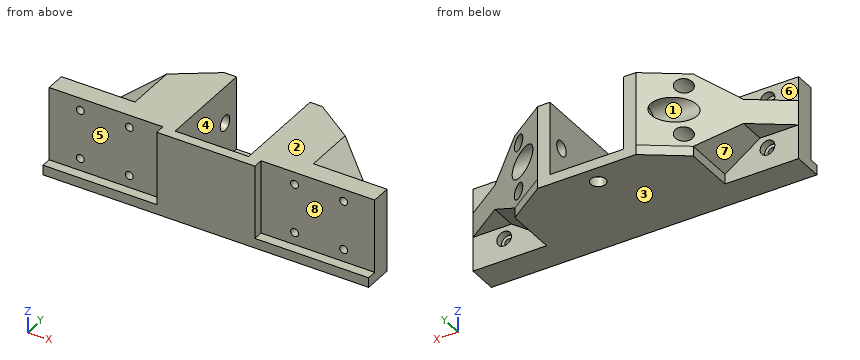
from build123d import *

# Parameters (mm, degrees)
SKETCH1_W               = 132.8
SKETCH1_H               = 44
BOSS_EXTRUDE1_DEPTH     = 4
SKETCH2_W               = 46.4
SKETCH2_H               = 8
BOSS_EXTRUDE2_DEPTH     = 30
BOSS_EXTRUDE3_DEPTH     = 15
CUT_EXTRUDE3_DEPTH      = 91.917325082
CUT_EXTRUDE3_DEPTH_BACK = 91.917325082
SKETCH6_R               = 3.1
SKETCH8_R               = 5.125
CUT_EXTRUDE5_DEPTH      = 96.419914064
SKETCH9_R               = 5.125
CUT_EXTRUDE6_DEPTH      = 96.419914064
CUT_EXTRUDE4_DEPTH      = 82.172409106
SKETCH3_R               = 1.6
CUT_EXTRUDE1_DEPTH      = 30
CUT_EXTRUDE2_DEPTH      = 82.172409106
CUT_EXTRUDE2_DEPTH_BACK = 3
SKETCH4_R               = 3
CUT_EXTRUDE7_DEPTH      = 77.11149716
SKETCH11_R              = 3.1
CUT_EXTRUDE8_DEPTH      = 77.11149716


with BuildPart() as part:
    # Sketch1 → Boss-Extrude1 (new body)
    with BuildSketch(Plane.XY):
        Rectangle(SKETCH1_W, SKETCH1_H)
    extrude(amount=BOSS_EXTRUDE1_DEPTH)

    # Sketch2 → Boss-Extrude2 (add)
    with BuildSketch(Plane.XY.offset(4)):
        with Locations((-43.2, -14)):
            Rectangle(SKETCH2_W, SKETCH2_H)
        Polygon((15, -18), (-15, -18), (-15, 22), (-20, 22), (-20, -10), (-20, -18), (-20, -22), (20, -22), (20, -18), (20, -10), (20, 22), (15, 22), align=None)
        with Locations((43.2, -14)):
            Rectangle(SKETCH2_W, SKETCH2_H)
    extrude(amount=BOSS_EXTRUDE2_DEPTH)

    # Sketch5 → Boss-Extrude3 (add, symmetric)
    with BuildSketch(Plane.XY.offset(19)):
        Polygon((20, -10), (66.4, -10), (20, 22), align=None)
        Polygon((-20, 22), (-20, -10), (-66.4, -10), align=None)
    extrude(amount=BOSS_EXTRUDE3_DEPTH, both=True)

    # Sketch6 → Cut-Extrude3 (cut, two sides: drawn at the far end of the back side and taken through both)
    with BuildSketch(Plane(origin=(-15, 0, 0), x_dir=(0, 0, -1), z_dir=(1, 0, 0)).offset(-CUT_EXTRUDE3_DEPTH_BACK)):
        with Locations(Location((-19, 14.5, 0), (0, 0, 90))):
            Circle(SKETCH6_R)
    extrude(amount=CUT_EXTRUDE3_DEPTH + CUT_EXTRUDE3_DEPTH_BACK, mode=Mode.SUBTRACT)

    # Sketch8 → Cut-Extrude5 (cut, through all)
    with BuildSketch(Plane(origin=(20, 0, 0), x_dir=(0, 0, -1), z_dir=(1, 0, 0))):
        with Locations(Location((-19, 14.5, 0), (0, 0, 90))):
            Circle(SKETCH8_R)
    extrude(amount=CUT_EXTRUDE5_DEPTH, mode=Mode.SUBTRACT)

    # Sketch9 → Cut-Extrude6 (cut, through all)
    with BuildSketch(Plane.ZY.offset(20)):
        with Locations(Location((19, 14.5, 0), (0, 0, 90))):
            Circle(SKETCH9_R)
    extrude(amount=CUT_EXTRUDE6_DEPTH, mode=Mode.SUBTRACT)

    # Sketch7 → Cut-Extrude4 (cut, through all)
    with BuildSketch(Plane(origin=(0, -10, 0), x_dir=(1, 0, 0), z_dir=(0, 1, 0))):
        Polygon((50.681480067, -14), (66.4, -14), (66.4, -4), (36.4, -4), align=None)
        Polygon((66.4, -34), (66.4, -24), (50.681480067, -24), (36.4, -34), align=None)
        Polygon((-66.4, -4), (-66.4, -14), (-50.681480067, -14), (-36.4, -4), align=None)
        Polygon((-50.681480067, -24), (-66.4, -24), (-66.4, -34), (-36.4, -34), align=None)
    extrude(amount=CUT_EXTRUDE4_DEPTH, mode=Mode.SUBTRACT)

    # Sketch3 → Cut-Extrude1 (cut)
    with BuildSketch(Plane(origin=(0, -10, 0), x_dir=(1, 0, 0), z_dir=(0, 1, 0))):
        with Locations(Location((-53.7, -9, 0), (0, 0, 270))):
            Circle(SKETCH3_R)
        with Locations(Location((-33.7, -29, 0), (0, 0, 270))):
            Circle(SKETCH3_R)
        with Locations(Location((-33.7, -9, 0), (0, 0, 270))):
            Circle(SKETCH3_R)
        with Locations(Location((-53.7, -29, 0), (0, 0, 270))):
            Circle(SKETCH3_R)
        with Locations(Location((33.7, -9, 0), (0, 0, 270))):
            Circle(SKETCH3_R)
        with Locations(Location((33.7, -29, 0), (0, 0, 270))):
            Circle(SKETCH3_R)
        with Locations(Location((53.7, -29, 0), (0, 0, 270))):
            Circle(SKETCH3_R)
        with Locations(Location((53.7, -9, 0), (0, 0, 270))):
            Circle(SKETCH3_R)
    extrude(amount=-CUT_EXTRUDE1_DEPTH, mode=Mode.SUBTRACT)

    # Sketch4 → Cut-Extrude2 (cut, two sides: drawn at the far end of the back side and taken through both)
    with BuildSketch(Plane(origin=(0, -10, 0), x_dir=(1, 0, 0), z_dir=(0, 1, 0)).offset(-CUT_EXTRUDE2_DEPTH_BACK)):
        with Locations(Location((-53.7, -9, 0), (0, 0, 90))):
            Circle(SKETCH4_R)
        with Locations(Location((-33.7, -9, 0), (0, 0, 180))):
            Circle(SKETCH4_R)
        with Locations(Location((-33.7, -29, 0), (0, 0, 180))):
            Circle(SKETCH4_R)
        with Locations(Location((-53.7, -29, 0), (0, 0, 270))):
            Circle(SKETCH4_R)
        with Locations((33.7, -9)):
            Circle(SKETCH4_R)
        with Locations(Location((53.7, -9, 0), (0, 0, 90))):
            Circle(SKETCH4_R)
        with Locations(Location((53.7, -29, 0), (0, 0, 90))):
            Circle(SKETCH4_R)
        with Locations((33.7, -29)):
            Circle(SKETCH4_R)
    extrude(amount=CUT_EXTRUDE2_DEPTH + CUT_EXTRUDE2_DEPTH_BACK, mode=Mode.SUBTRACT)

    # Sketch10 → Cut-Extrude7 (cut, through all)
    with BuildSketch(Plane.XY.offset(4)):
        Polygon((20, 22), (36.4, 10.689655172), (36.4, -10), (66.4, -10), (66.4, 22), align=None)
        Polygon((-66.4, 22), (-20, 22), (-36.4, 10.689655172), (-36.4, -10), (-66.4, -10), align=None)
    extrude(amount=-CUT_EXTRUDE7_DEPTH, mode=Mode.SUBTRACT)

    # Sketch11 → Cut-Extrude8 (cut, through all)
    with BuildSketch(Plane.XY.offset(4)):
        with Locations((0, 14.5)):
            Circle(SKETCH11_R)
    extrude(amount=-CUT_EXTRUDE8_DEPTH, mode=Mode.SUBTRACT)


solid = part.part
Source: CAD feature listing. Evaluate the final solid. Frame: model axes, mm. Face numbers are marked on the shaded views. A direction names the side the tool comes from. Coordinates: 2 decimals unless noted, no trailing zeros. Write each loop counter-clockwise with the first axis right and the second up, starting at its lowest first coordinate (ties: lowest second). Pieces come first, ordered by that corner, then holes. Notation, with made-up numbers: M 42.25,-22.75 L 67.25,-22.75 A24 ccw 67.25,11.25 Z; hole C 38,58 d9. An arc over 180 degrees is marked long. Use a Markdown table: item, result.
1) Mould query, pull axis Z, two halves, no side actions, for the marked faces 1, 2, 3 and 4. Classes: pulls with the +Z half, pulls with the -Z half, needs draft (parallel to the pull), parting line crosses it, or undercut.
Conclusion:
| item | result |
|---|---|
| face 1 | undercut |
| face 2 | pulls with the +Z half |
| face 3 | pulls with the -Z half |
| face 4 | needs draft |
2) First-contact query: pin 1 Ø3 at (y, z) = (16.5, 4) entering from -X; pin 2 Ø3.5 at (x, z) = (-33.7, 9) entering from -Y; pin 3 Ø1.8 at (x, z) = (33, 8) entering from +Y. Flat tips, straight axial feed; report the tip coordinate or a pass-through.
Conclusion:
| item | result |
|---|---|
| pin 1 | stops at x = -30.15 |
| pin 2 | stops at y = -18 |
| pin 3 | stops at y = -13 |
3) Section B-B, the plane y = -4.5. Output: boundary loops of the cut face in (x, z) (3 decimals), then the cut area to 3 significant figures.
Conclusion:
| item | result |
|---|---|
| outline | M -58.425,14 L -50.681,14 L -36.4,4 L -36.4,0 L 36.4,0 L 36.4,4 L 50.681,14 L 58.425,14 L 58.425,24 L 50.681,24 L 36.4,34 L 15,34 L 15,4 L -15,4 L -15,34 L -36.4,34 L -50.681,24 L -58.425,24 Z; hole C -33.7,9 d6; hole C -33.7,29 d6; hole C 33.7,9 d6; hole C 33.7,29 d6 |
| area | 2,190 mm^2 |
4) Section D-D, the plane z = 29. Give the number of separate pieces and of enclosed holes in the cut face, then the cut area to 3 significant figures.
Conclusion:
| item | result |
|---|---|
| separate pieces | 5 |
| enclosed holes | 0 |
| area | 2,020 mm^2 |
5) Reachability of the marked faces 5, 6, 7 and 8 from +Z, -Z, +X, -X, +Y, -Y: full face, straight path, thin tool, end or side. Return the list, or none.
Conclusion:
| item | result |
|---|---|
| face 5 | +Z, -X, -Y |
| face 6 | +Z, -X, +Y |
| face 7 | -Z, -X, +Y |
| face 8 | +Z, +X, -Y |
6) Section C-C, the plane x = -53.7. Output: boundary loops of the cut face in (y, z), then the cut area to 3 significant figures.
Conclusion:
| item | result |
|---|---|
| outline | M -22,0 L -10,0 L -10,6 L -13,6 L -13,7.4 L -18,7.4 L -18,4 L -22,4 Z; M -18,10.6 L -13,10.6 L -13,12 L -10,12 L -10,14 L -1.24,14 L -1.24,24 L -10,24 L -10,26 L -13,26 L -13,27.4 L -18,27.4 Z; M -18,30.6 L -13,30.6 L -13,32 L -10,32 L -10,34 L -18,34 Z |
| area | 308 mm^2 |
7) Ray query, L1, parallel to X at y = -14.35, z = 29; L2, parallel to X at y = 1, z = 9; L3, parallel to Z at x = 33, y = -14.5. Return the intervals inside material, ascending.
Conclusion:
| item | result |
|---|---|
| L1 | x = -66.4 to -55.3, -52.1 to -35.3, -32.1 to -15, 15 to 32.1, 35.3 to 52.1, 55.3 to 66.4 |
| L2 | x = -43.54 to -36.7, -30.7 to -15, 15 to 30.7, 36.7 to 43.54 |
| L3 | z = 0 to 7.56, 10.44 to 27.56, 30.44 to 34 |
8) Section A-A, the plane x = 0. Output: boundary loops of the cut face in (y, z), then the cut area to 3 significant figures.
Conclusion:
| item | result |
|---|---|
| outline | M -22,0 L 11.4,0 L 11.4,4 L -18,4 L -18,34 L -22,34 Z; M 17.6,0 L 22,0 L 22,4 L 17.6,4 Z |
| area | 271 mm^2 |
